```python
from build123d import *

# Parameters (mm, degrees)
F1_DEPTH = 5.08
F2_R     = 4


# Not quite as in the source:
# - a feature names something its author has since deleted; it is built from what else it names


with BuildPart() as f1:
    # F0 (on Top) → F1 (new body)
    with BuildSketch(Plane.XY):
        with BuildLine():
            Line((0.6656670719, 55.2782733088), (-50.5843329281, 55.2782733088))
            ThreePointArc((-50.5843329281, 55.2782733088), (-50.7887088575, 54.5223908657), (-51.3461439517, 53.9724873251))
            Line((-51.3461439517, 53.9724873251), (-49.5403858838, 50.7782733088))
            Line((-49.5403858838, 50.7782733088), (-11.5572661318, 50.7782733088))
            Line((-11.5572661318, 50.7782733088), (-3.4960969558, 50.7782733088))
            Line((-3.4960969558, 50.7782733088), (5.4156670719, 50.7782733088))
            Line((5.4156670719, 50.7782733088), (10.9156670719, 50.7782733088))
            Line((10.9156670719, 50.7782733088), (10.9156670719, 55.2782733088))
            Line((10.9156670719, 55.2782733088), (3.6656670719, 55.2782733088))
            ThreePointArc((3.6656670719, 55.2782733088), (2.1656670719, 53.7782733088), (0.6656670719, 55.2782733088))
        make_face()
        with BuildLine():
            Line((-11.5572661318, 4.5), (-23.3782799724, 4.5))
            Line((-23.3782799724, 4.5), (-21.5725219045, 1.3057859837))
            ThreePointArc((-21.5725219045, 1.3057859837), (-20.0784504851, 1.2956240706), (-19.3343329281, 0))
            Line((-19.3343329281, 0), (10.9156670719, 0))
            Line((10.9156670719, 0), (10.9156670719, 4.5))
            Line((10.9156670719, 4.5), (5.4156670719, 4.5))
            Line((5.4156670719, 4.5), (-3.4960969558, 4.5))
            Line((-3.4960969558, 4.5), (-11.5572661318, 4.5))
        make_face()
        with BuildLine():
            ThreePointArc((-51.3461439517, 53.9724873251), (-53.3799569987, 56.0341557518), (-50.5843329281, 55.2782733088))
            Line((-50.5843329281, 55.2782733088), (0.6656670719, 55.2782733088))
            ThreePointArc((0.6656670719, 55.2782733088), (2.1656670719, 56.7782733088), (3.6656670719, 55.2782733088))
            Line((3.6656670719, 55.2782733088), (10.9156670719, 55.2782733088))
            Line((10.9156670719, 55.2782733088), (18.1656670719, 55.2782733088))
            ThreePointArc((18.1656670719, 55.2782733088), (19.6656670719, 56.7782733088), (21.1656670719, 55.2782733088))
            Line((21.1656670719, 55.2782733088), (28.1048402488, 55.2782733088))
            Line((28.1048402488, 55.2782733088), (28.1048402488, 57.7362733088))
            Line((28.1048402488, 57.7362733088), (31.2798402488, 57.7362733088))
            Line((31.2798402488, 57.7362733088), (31.2798402488, 55.2782733088))
            Line((31.2798402488, 55.2782733088), (39.3168402488, 55.2782733088))
            Line((39.3168402488, 55.2782733088), (39.3168402488, 57.7362733088))
            Line((39.3168402488, 57.7362733088), (42.4918402488, 57.7362733088))
            Line((42.4918402488, 57.7362733088), (42.4918402488, 55.2782733088))
            Line((42.4918402488, 55.2782733088), (71.6656670719, 55.2782733088))
            ThreePointArc((71.6656670719, 55.2782733088), (73.9156670719, 57.5282733088), (76.1656670719, 55.2782733088))
            ThreePointArc((76.1656670719, 55.2782733088), (75.0494907365, 53.3348372029), (72.8083836073, 53.3195943333))
            Line((72.8083836073, 53.3195943333), (71.3717200276, 50.7782733088))
            Line((71.3717200276, 50.7782733088), (81.8841302488, 50.7782733088))
            Line((81.8841302488, 50.7782733088), (81.8841302488, 59.7782733088))
            Line((81.8841302488, 59.7782733088), (-60.052796105, 59.7782733088))
            Line((-60.052796105, 59.7782733088), (-60.052796105, 50.7782733088))
            Line((-60.052796105, 50.7782733088), (-49.5403858838, 50.7782733088))
            Line((-49.5403858838, 50.7782733088), (-51.3461439517, 53.9724873251))
        make_face()
        with BuildLine():
            Line((-21.5725219045, 1.3057859837), (-23.3782799724, 4.5))
            Line((-23.3782799724, 4.5), (-27.3365851734, 4.5))
            Line((-27.3365851734, 4.5), (-27.3365851734, -4.5))
            Line((-27.3365851734, -4.5), (49.1679193172, -4.5))
            Line((49.1679193172, -4.5), (49.1679193172, 4.5))
            Line((49.1679193172, 4.5), (45.2096141162, 4.5))
            Line((45.2096141162, 4.5), (43.4038560483, 1.3057859837))
            ThreePointArc((43.4038560483, 1.3057859837), (43.9612911425, 0.7558824431), (44.1656670719, 0))
            ThreePointArc((44.1656670719, 0), (42.6656670719, -1.5), (41.1656670719, 0))
            Line((41.1656670719, 0), (31.6349193172, 0))
            Line((31.6349193172, 0), (31.6349193172, -2.5))
            Line((31.6349193172, -2.5), (28.4599193172, -2.5))
            Line((28.4599193172, -2.5), (28.4599193172, 0))
            Line((28.4599193172, 0), (20.3669193172, 0))
            Line((20.3669193172, 0), (20.3669193172, -2.5))
            Line((20.3669193172, -2.5), (17.1919193172, -2.5))
            Line((17.1919193172, -2.5), (17.1919193172, 0))
            Line((17.1919193172, 0), (10.9156670719, 0))
            Line((10.9156670719, 0), (-19.3343329281, 0))
            ThreePointArc((-19.3343329281, 0), (-21.5902153712, -1.2956240706), (-21.5725219045, 1.3057859837))
        make_face()
        with BuildLine():
            Line((10.9156670719, 4.5), (10.9156670719, 0))
            Line((10.9156670719, 0), (17.1919193172, 0))
            Line((17.1919193172, 0), (17.1919193172, 2.5))
            Line((17.1919193172, 2.5), (20.3669193172, 2.5))
            Line((20.3669193172, 2.5), (20.3669193172, 0))
            Line((20.3669193172, 0), (28.4599193172, 0))
            Line((28.4599193172, 0), (28.4599193172, 2.5))
            Line((28.4599193172, 2.5), (31.6349193172, 2.5))
            Line((31.6349193172, 2.5), (31.6349193172, 0))
            Line((31.6349193172, 0), (41.1656670719, 0))
            ThreePointArc((41.1656670719, 0), (41.9097846288, 1.2956240706), (43.4038560483, 1.3057859837))
            Line((43.4038560483, 1.3057859837), (45.2096141162, 4.5))
            Line((45.2096141162, 4.5), (33.3886002756, 4.5))
            Line((33.3886002756, 4.5), (25.3274310996, 4.5))
            Line((25.3274310996, 4.5), (16.4156670719, 4.5))
            Line((16.4156670719, 4.5), (10.9156670719, 4.5))
        make_face()
        with BuildLine():
            Line((18.1656670719, 55.2782733088), (10.9156670719, 55.2782733088))
            Line((10.9156670719, 55.2782733088), (10.9156670719, 50.7782733088))
            Line((10.9156670719, 50.7782733088), (16.4156670719, 50.7782733088))
            Line((16.4156670719, 50.7782733088), (25.3274310996, 50.7782733088))
            Line((25.3274310996, 50.7782733088), (33.3886002756, 50.7782733088))
            Line((33.3886002756, 50.7782733088), (71.3717200276, 50.7782733088))
            Line((71.3717200276, 50.7782733088), (72.8083836073, 53.3195943333))
            ThreePointArc((72.8083836073, 53.3195943333), (71.972230966, 54.1444496442), (71.6656670719, 55.2782733088))
            Line((71.6656670719, 55.2782733088), (42.4918402488, 55.2782733088))
            Line((42.4918402488, 55.2782733088), (42.4918402488, 52.7362733088))
            Line((42.4918402488, 52.7362733088), (39.3168402488, 52.7362733088))
            Line((39.3168402488, 52.7362733088), (39.3168402488, 55.2782733088))
            Line((39.3168402488, 55.2782733088), (31.2798402488, 55.2782733088))
            Line((31.2798402488, 55.2782733088), (31.2798402488, 52.7362733088))
            Line((31.2798402488, 52.7362733088), (28.1048402488, 52.7362733088))
            Line((28.1048402488, 52.7362733088), (28.1048402488, 55.2782733088))
            Line((28.1048402488, 55.2782733088), (21.1656670719, 55.2782733088))
            ThreePointArc((21.1656670719, 55.2782733088), (19.6656670719, 53.7782733088), (18.1656670719, 55.2782733088))
        make_face()
        Polygon((5.4156670719, 38.6288985841), (5.4156670719, 27.6391366544), (10.9156670719, 27.6391366544), (10.9156670719, 50.7782733088), (5.4156670719, 50.7782733088), align=None)
        Polygon((10.9156670719, 27.6391366544), (5.4156670719, 27.6391366544), (5.4156670719, 16.6493747247), (5.4156670719, 4.5), (10.9156670719, 4.5), align=None)
        Polygon((16.4156670719, 50.7782733088), (10.9156670719, 50.7782733088), (10.9156670719, 27.6391366544), (16.4156670719, 27.6391366544), (16.4156670719, 38.6288985841), align=None)
        Polygon((16.4156670719, 27.6391366544), (10.9156670719, 27.6391366544), (10.9156670719, 4.5), (16.4156670719, 4.5), (16.4156670719, 16.6493747247), align=None)
        Polygon((-3.4960969558, 50.7782733088), (-11.5572661318, 50.7782733088), (5.4156670719, 27.6391366544), (5.4156670719, 38.6288985841), align=None)
        Polygon((5.4156670719, 27.6391366544), (-11.5572661318, 4.5), (-3.4960969558, 4.5), (5.4156670719, 16.6493747247), align=None)
        Polygon((33.3886002756, 4.5), (16.4156670719, 27.6391366544), (16.4156670719, 16.6493747247), (25.3274310996, 4.5), align=None)
        Polygon((16.4156670719, 38.6288985841), (16.4156670719, 27.6391366544), (33.3886002756, 50.7782733088), (25.3274310996, 50.7782733088), align=None)
    extrude(amount=F1_DEPTH)

    # F2
    f2_edges = [f1.edges().sort_by_distance(p)[0] for p in [
        (-60.052796, 59.778273, 2.54),
        (-60.052796, 50.778273, 2.54),
        (81.88413, 59.778273, 2.54),
        (81.88413, 50.778273, 2.54),
        (49.167919, 4.5, 2.54),
        (49.167919, -4.5, 2.54),
        (-27.336585, 4.5, 2.54),
        (-27.336585, -4.5, 2.54),
    ]]
    fillet(f2_edges, radius=F2_R)


solid = f1.part
```
CAD build for the part. Positions are in the model's coordinates, mm. A direction names the side the tool comes from. Round coordinates to 2 decimals unless told otherwise and drop trailing zeros. Order: outer loops, then holes, each group sorted by start corner. A loop starts at its lowest first (then second) coordinate and runs counter-clockwise, first axis right, second up. Notation, with made-up numbers: (81.25, -7) -> (140.25, -7) arc R23 cw to (140.25, 1) -> close; hole circle Ø8 at (34.5, 63). An arc over 180 degrees is marked (long way). Write item = value, one per line.
(1) Cut at B-B (x = 23). Write the cut outline in (y, z).
Answers follow:
outline = (-4.5, 0) -> (4.5, 0) -> (4.5, 5.08) -> (-4.5, 5.08) -> close; (7.67, 0) -> (18.66, 0) -> (18.66, 5.08) -> (7.67, 5.08) -> close; (36.62, 0) -> (47.61, 0) -> (47.61, 5.08) -> (36.62, 5.08) -> close; (50.78, 0) -> (59.78, 0) -> (59.78, 5.08) -> (50.78, 5.08) -> close
(2) Cut at A-A (y = 14.5). Write the cut outline in (x, z).
Answers follow:
outline = (-4.22, 0) -> (3.84, 0) -> (3.84, 5.08) -> (-4.22, 5.08) -> close; (5.42, 0) -> (16.42, 0) -> (16.42, 5.08) -> (5.42, 5.08) -> close; (17.99, 0) -> (26.05, 0) -> (26.05, 5.08) -> (17.99, 5.08) -> close
(3) 3-axis set-ups, long thin cutter, end or side, ignore diameter. For faces 1 (the flat face through (55, 50.778, 3)), 2 (the cylindrical face through (-26.134, 3.359, 2.576)), 3 (the flat face through (39.317, 55, 3)): which of +Z, -Z, +X, -X, +Y, -Y reach the whole face in a straight line?
Answers follow:
face_1 = +Z, -Z, +X
face_2 = +Z, -Z, -X
face_3 = +Z, -Z
(4) Pull direction X, two halves, no side cores. Call faces 4 (the cylindrical face through (-58.85, 58.64, 2.58)), 5 (the cylindrical face through (47.965, -3.359, 2.576)), 6 (the flat face through (21, 50.778, 3)): +X half, -X half, draft (parallel to the pull), parting line (faces both ways), or undercut.
Answers follow:
face_4 = -X half
face_5 = +X half
face_6 = undercut
(5) Drill centre lines: L1, parallel to Y at x = -52, z = 0.4; L2, parallel to Y at x = -15, z = 3.3; L3, parallel to X at y = -1, z = 3.1. Where is each one in solid material? Low to high.
Answers follow:
L1 = 50.78 to 53.78, 56.78 to 59.78
L2 = -4.5 to 4.5, 50.78 to 59.78
L3 = -27.31 to -21.95, -19.72 to 17.19, 20.37 to 28.46, 31.63 to 41.55, 43.78 to 49.14
(6) Cut at C-C (z = 2.1). State how many separate pieces and enclosed holes the cut face has, plus the area to 3 significant figures.
Answers follow:
separate_pieces = 1
enclosed_holes = 14
area = 2,900 mm²
(7) Flat gauge pins, fed straight in: P1, Ø1.5, axis at x = -25.5, z = 2.5, coming from the -Y side; P2, Ø1.5, axis at y = 0.5, z = 2, coming from the -X side; P3, Ø5, axis at x = 2.17, y = 55.28, coming from the -Z side. Where does each tip first touch, or does it go through?
Answers follow:
P1 = -4.24
P2 = -27.34
P3 = 0
(8) Cut at D-D (x = -36). Write the cut outline in (y, z).
Answers follow:
outline = (50.78, 0) -> (59.78, 0) -> (59.78, 5.08) -> (50.78, 5.08) -> close
